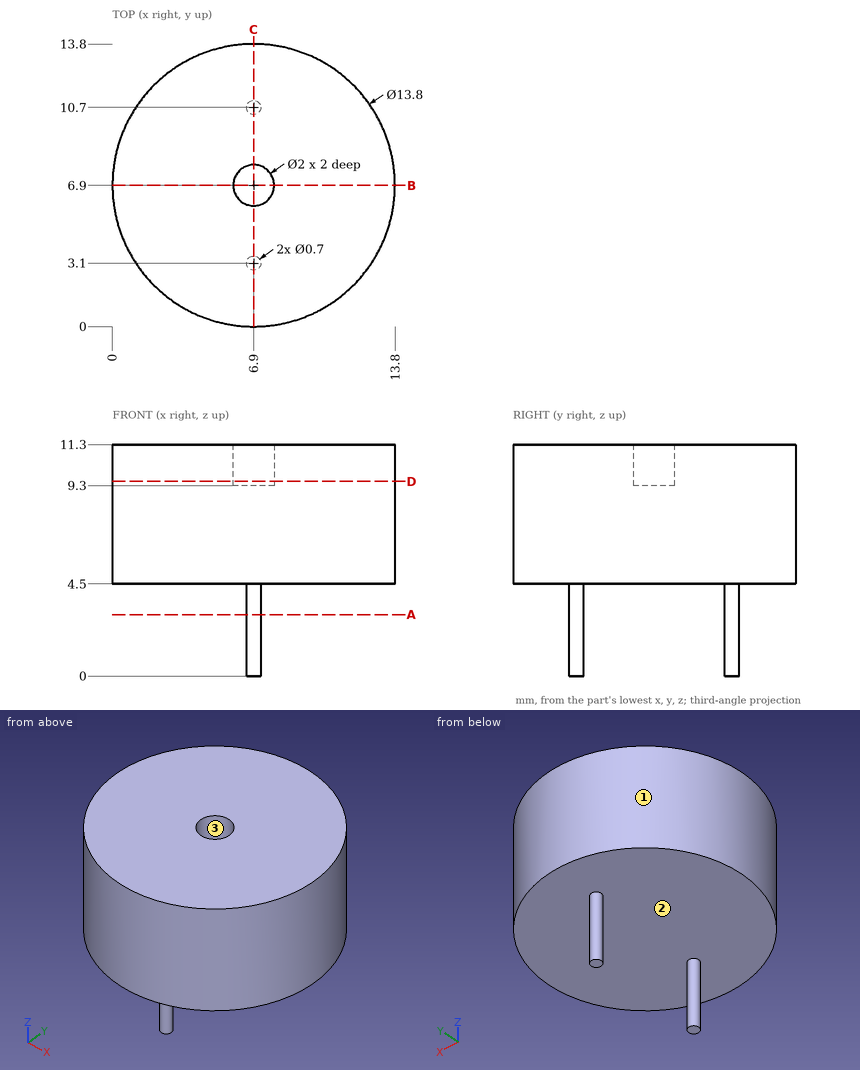
Answer from the drawing. Dimensions are ordinates in mm from the lowest x, y and z of the part. Round coordinates to 2 decimals unless told otherwise and drop trailing zeros. Order: outer loops, then holes, each group sorted by start corner. A loop starts at its lowest first (then second) coordinate and runs counter-clockwise, first axis right, second up. Notation, with made-up numbers: (58.5, 42.5) - (117.5, 42.5) arc R10 cw to (117.5, 58.5) - close; hole circle Ø2 at (46, 43). An arc over 180 degrees is marked (long way). Put each result on its own line as item: value. Start each with the question number.
(1) Find section B-B (y = 6.9). Give the vertices of the cut face in (x, z).
(2) Find section C-C (x = 6.9). Give the vertices of the cut face in (y, z).
(3) Find section D-D (z = 9.5). Give the vertices of the cut face in (x, y).
(4) Straight lines are drawn through the part: probe 1 along Y at (x, z) = (6.9, 10.6); probe 2 along Z at (x, y) = (11.5, 9.5); probe 3 along X at (y, z) = (10.5, 6.5). For each, find the intervals that lie inside material, in ascending order. Write a range as from..to.
(5) Find section A-A (z = 3). Give the vertices of the cut face in (x, y), plus the area to 3 significant figures.
(6) Given P1, Ø1, axis at x = 10, y = 9.5, coming from the -Z side; P2, Ø5, axis at x = 10, z = 5, coming from the -Y side; P3, Ø4, axis at y = 2, z = 3, coming from the -X side, each flat-ended and moving along its own axis, determine where each tip first touches the part or whether it passes through.
(7) Determine the mould class of the marked faces 1, 2 and 3 for opening direction X: released by +X, released by -X, zero draft, split by the parting line, or undercut.
Reply:
1. outline: (0, 4.5) - (13.8, 4.5) - (13.8, 11.3) - (7.9, 11.3) - (7.9, 9.3) - (5.9, 9.3) - (5.9, 11.3) - (0, 11.3) - close
2. outline: (0, 4.5) - (2.75, 4.5) - (2.75, 0) - (3.45, 0) - (3.45, 4.5) - (10.35, 4.5) - (10.35, 0) - (11.05, 0) - (11.05, 4.5) - (13.8, 4.5) - (13.8, 11.3) - (7.9, 11.3) - (7.9, 9.3) - (5.9, 9.3) - (5.9, 11.3) - (0, 11.3) - close
3. outline: circle Ø13.8 at (6.9, 6.9); hole circle Ø2 at (6.9, 6.9)
4. probe 1: 0..5.9, 7.9..13.8
4. probe 2: 4.5..11.3
4. probe 3: 1.01..12.79
5. outline: circle Ø0.7 at (6.9, 3.1); circle Ø0.7 at (6.9, 10.7)
5. area: 0.770 mm^2
6. P1: z = 4.5
6. P2: y = 0.03
6. P3: x = 1
7. face 1: split by the parting line
7. face 2: zero draft
7. face 3: undercut
